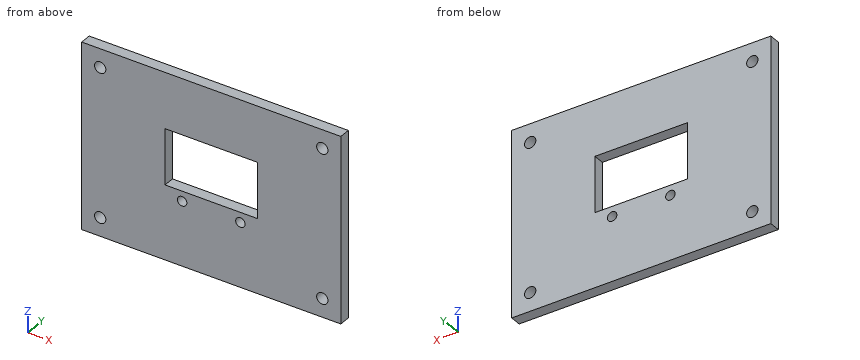
```python
from build123d import *

# Parameters (mm, degrees)
SKETCH1_W           = 70
SKETCH1_H           = 50
BOSS_EXTRUDE1_DEPTH = 3
SKETCH2_R           = 1.275
SKETCH2_W           = 25
SKETCH2_H           = 15
CUT_EXTRUDE1_DEPTH  = 3
SKETCH3_R           = 1.525
CUT_EXTRUDE2_DEPTH  = 3


with BuildPart() as part:
    # Sketch1 → Boss-Extrude1 (new body)
    with BuildSketch(Plane(origin=(0, 0, 0), x_dir=(1, 0, 0), z_dir=(0, 1, 0))):
        with Locations((35, 25)):
            Rectangle(SKETCH1_W, SKETCH1_H)
    extrude(amount=BOSS_EXTRUDE1_DEPTH)

    # Sketch2 → Cut-Extrude1 (cut)
    with BuildSketch(Plane(origin=(0, 3, 0), x_dir=(1, 0, 0), z_dir=(0, 1, 0))):
        with Locations(Location((27.135, 32.7, 0), (0, 0, 270))):
            Circle(SKETCH2_R)
        with Locations(Location((42.865, 32.7, 0), (0, 0, 90))):
            Circle(SKETCH2_R)
        with Locations((35, 22.5)):
            Rectangle(SKETCH2_W, SKETCH2_H)
    extrude(amount=-CUT_EXTRUDE1_DEPTH, mode=Mode.SUBTRACT)

    # Sketch3 → Cut-Extrude2 (cut)
    with BuildSketch(Plane(origin=(0, 3, 0), x_dir=(1, 0, 0), z_dir=(0, 1, 0))):
        with Locations(Location((5, 45, 0), (0, 0, 270))):
            Circle(SKETCH3_R)
        with Locations(Location((65, 45, 0), (0, 0, 90))):
            Circle(SKETCH3_R)
        with Locations(Location((65, 5, 0), (0, 0, 270))):
            Circle(SKETCH3_R)
        with Locations(Location((5, 5, 0), (0, 0, 90))):
            Circle(SKETCH3_R)
    extrude(amount=-CUT_EXTRUDE2_DEPTH, mode=Mode.SUBTRACT)


solid = part.part
```
Part model, mm, in its own coordinate system. Round coordinates to 2 decimals unless told otherwise and drop trailing zeros. Order: outer loops, then holes, each group sorted by start corner. A loop starts at its lowest first (then second) coordinate and runs counter-clockwise, first axis right, second up. Notation, with made-up numbers: M 26.5,46.5 L 55.5,46.5 A7 cw 55.5,54.5 Z; hole C 43.5,37.25 d1. An arc over 180 degrees is marked long. Put each result on its own line as item: value. Start each with the question number.
1. Slice it at C-C on z = -20. List the corners of the cut face in (x, y).
2. Slice it at B-B on x = 65. List the corners of the cut face in (y, z) (3 decimals), then the cut area to 3 significant figures.
3. Drill centre lines: probe 1 along X at (y, z) = (0.9, -45) (3 decimals); probe 2 along X at (y, z) = (1.65, -32.7); probe 3 along Z at (x, y) = (65, 1.7) (3 decimals). Where is each one in solid material? Low to high. Write a range as [from, to].
4. Drop a flat-ended pin along its axis: pin 1 (2.5 mm diameter, centred on x = 65, z = -5, fed in from +Y). Give the stop position or say it passes through.
5. Slice it at D-D on y = 1.35. List the corners of the cut face in (x, z) (3 decimals).
6. Slice it at A-A on z = -5. List the corners of the cut face in (x, y) (3 decimals).
Findings:
1. outline: M 0,0 L 22.5,0 L 22.5,3 L 0,3 Z; M 47.5,0 L 70,0 L 70,3 L 47.5,3 Z
2. outline: M 0,-50 L 3,-50 L 3,-46.525 L 0,-46.525 Z; M 0,-43.475 L 3,-43.475 L 3,-6.525 L 0,-6.525 Z; M 0,-3.475 L 3,-3.475 L 3,0 L 0,0 Z
2. area: 132 mm2
3. probe 1: [0, 3.475], [6.525, 63.475], [66.525, 70]
3. probe 2: [0, 25.86], [28.41, 41.59], [44.14, 70]
3. probe 3: [-50, -46.525], [-43.475, -6.525], [-3.475, 0]
4. pin 1: through
5. outline: M 0,-50 L 70,-50 L 70,0 L 0,0 Z; hole C 5,-45 d3.05; hole C 5,-5 d3.05; hole M 22.5,-30 L 47.5,-30 L 47.5,-15 L 22.5,-15 Z; hole C 27.135,-32.7 d2.55; hole C 42.865,-32.7 d2.55; hole C 65,-45 d3.05; hole C 65,-5 d3.05
6. outline: M 0,0 L 3.475,0 L 3.475,3 L 0,3 Z; M 6.525,0 L 63.475,0 L 63.475,3 L 6.525,3 Z; M 66.525,0 L 70,0 L 70,3 L 66.525,3 Z
